Drawing for the job (mm, zero at the part's lowest x, y, z). A direction names the side the tool comes from. Round coordinates to 2 decimals unless told otherwise and drop trailing zeros. Loops run counter-clockwise (first coordinate to the right, second up) from the corner with the lowest first, then second, coordinate; pieces in that order, holes last. Notation, with made-up numbers: M -17.5,-21 L -13.5,-21 A23 cw -13.5,14 Z; hole C 72,-3 d4. An arc over 180 degrees is marked long. Use a Markdown table: item, result. Add a question column.
Q1. Probe line 1 (X direction, y = 3.25, z = 9.5) (1 decimal); line 2 (X direction, y = 12.75, z = 9.5); line 3 (Z direction, x = 15, y = 13.75) (1 decimal). List the from-to ranges inside material, lowest first. Write a range as from..to.
Q2. Pin check, flat tip, straight feed: pin 1 (3 mm diameter, centred on x = 15.5, z = 8.5, fed in from +Y). Stop position of the tip, or through.
Q3. Cut at B-B (z = 9.5). Give the cut face in (x, y) (1 decimal), plus the area to 3 significant figures.
Q4. Tool access for the marked faces 1 and 2: list every direction of +Z, -Z, +X, -X, +Y, -Y with a clear straight run to the whole face (end or side of a thin tool).
Q5. Cut at D-D (z = 2.5). Give the cut face in (x, y) (1 decimal).
Q6. Cut at A-A (y = 8.75). State how many separate pieces and enclosed holes the cut face has.
Q7. Mould opens along X. For the marked faces 3, 4 and 5 say: +X half, -X half, draft (parallel to the pull), parting line (faces both ways), or undercut.
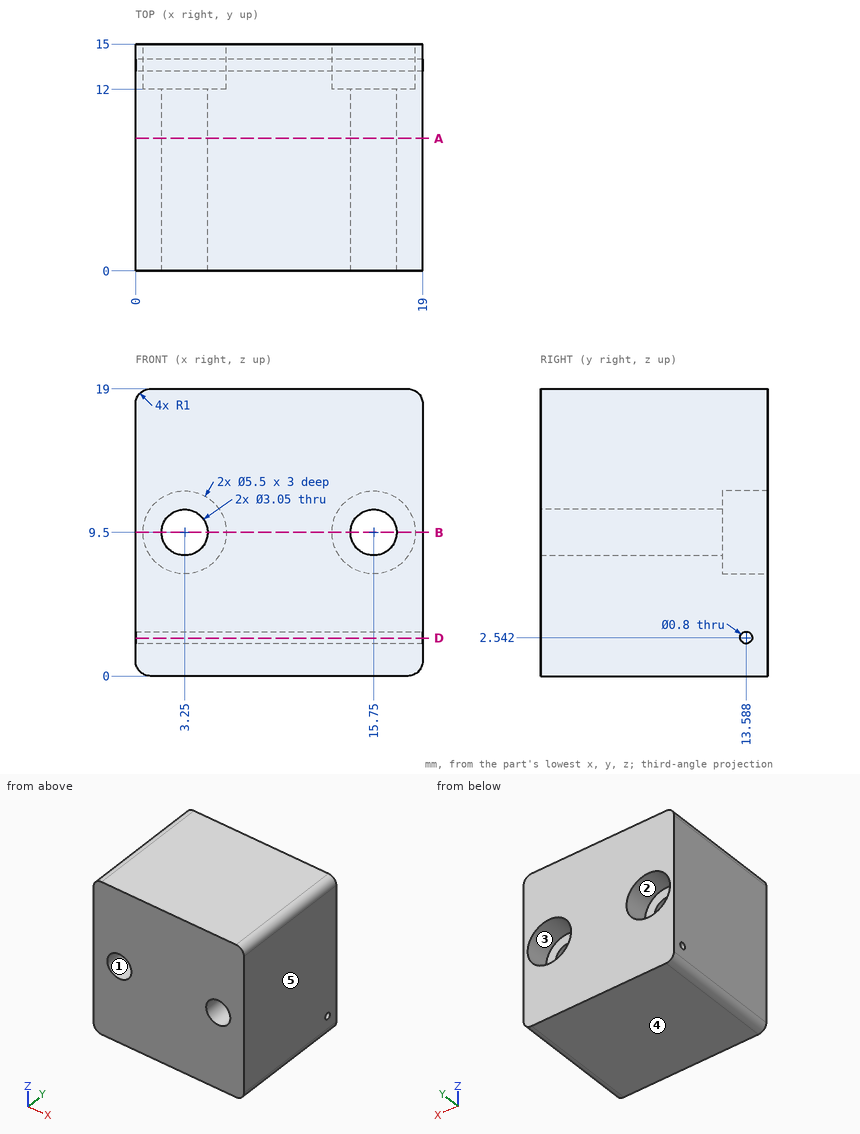
Checked values:
| question | item | result |
|---|---|---|
| 1 | line 1 | x = 0..1.7, 4.8..14.2, 17.3..19 |
| 1 | line 2 | x = 0..0.5, 6..13, 18.5..19 |
| 1 | line 3 | z = 0..2.2, 2.9..6.9, 12.1..19 |
| 2 | pin 1 | stops at y = 12 |
| 3 | outline | M 0,0 L 1.7,0 L 1.7,12 L 0.5,12 L 0.5,15 L 0,15 Z; M 4.8,0 L 14.2,0 L 14.2,12 L 13,12 L 13,15 L 6,15 L 6,12 L 4.8,12 Z; M 17.3,0 L 19,0 L 19,15 L 18.5,15 L 18.5,12 L 17.3,12 Z |
| 3 | area | 179 mm^2 |
| 4 | face 1 | +Y, -Y |
| 4 | face 2 | +Y |
| 5 | outline | M 0,0 L 19,0 L 19,13.2 L 0,13.2 Z; M 0,14 L 19,14 L 19,15 L 0,15 Z |
| 6 | separate pieces | 1 |
| 6 | enclosed holes | 2 |
| 7 | face 3 | undercut |
| 7 | face 4 | draft |
| 7 | face 5 | +X half |
